Autodesk Inventor part; units mm, degrees
ref_plane "YZ Plane" through (0, 0, 0) normal (1, 0, 0) x (0, 1, 0)
ref_plane "XZ Plane" through (0, 0, 0) normal (0, 1, 0) x (-1, 0, 0)
ref_plane "XY Plane" through (0, 0, 0) normal (0, 0, 1) x (1, 0, 0)
sketch "Sketch1" plane through (0, 0, 0) normal (0, 0, 1) x (1, 0, 0)
  line L0 (0, 0) -> (139.7, 0)
  line L1 (139.7, 0) -> (139.7, 76.2)
  line L2 (139.7, 76.2) -> (0, 76.2)
  line L3 (0, 76.2) -> (0, 0)
  dimension "d0" = 139.7
  dimension "d1" = 76.2
extrude "Extrusion1" add sketch "Sketch1" along normal blind 3.175
sketch "Sketch2" plane through (0, 0, 3.175) normal (0, 0, 1) x (1, 0, 0)
  line L0 (0, 0) -> (139.7, 0)
  line L1 (139.7, 0) -> (139.7, 76.2)
  line L2 (139.7, 76.2) -> (0, 76.2)
  line L3 (0, 76.2) -> (0, 0)
  circle A0 centre (6.35, 69.85) radius 2.54
  circle A1 centre (6.35, 6.35) radius 2.54
  circle A2 centre (133.35, 6.35) radius 2.54
  circle A3 centre (133.35, 69.85) radius 2.54
  circle A4 centre (63.5, 38.1) radius 11.1125
  circle A5 centre (104.14, 38.1) radius 14.2875
  dimension "d4" = 6.35
  dimension "d5" = 6.35
  dimension "d6" = 69.85
  dimension "d7" = 6.35
  dimension "d8" = 133.35
  dimension "d9" = 6.35
  dimension "d10" = 133.35
  dimension "d11" = 69.85
  dimension "d12" = 63.5
  dimension "d13" = 38.1
  dimension "d14" = 38.1
  dimension "d15" = 104.14
  dimension "d16" = 5.08
  dimension "d17" = 5.08
  dimension "d18" = 5.08
  dimension "d19" = 5.08
  dimension "d20" = 22.225
  dimension "d21" = 28.575
extrude "Extrusion2" cut sketch "Sketch2" against normal blind 3.175 contours A0 | A1 | A2 | A3 | A4 | A5
sketch "Sketch3" plane through (0, 0, 3.175) normal (0, 0, 1) x (1, 0, 0)
  circle A0 centre (63.5, 38.1) radius 11.1125
  circle A1 centre (133.35, 6.35) radius 2.54
  circle A2 centre (6.35, 69.85) radius 2.54
  circle A3 centre (6.35, 6.35) radius 2.54
  circle A4 centre (133.35, 69.85) radius 2.54
  circle A5 centre (104.14, 38.1) radius 14.2875
  line L0 (0, 0) -> (139.7, 0)
  line L1 (139.7, 0) -> (139.7, 76.2)
  line L2 (139.7, 76.2) -> (0, 76.2)
  line L3 (0, 76.2) -> (0, 0)
  line L4 (0, 76.2) -> (0, 0)
  line L5 (0, 25.4) -> (-25.4, 25.4)
  line L6 (-25.4, 25.4) -> (-25.4, 50.8)
  line L7 (-25.4, 50.8) -> (0, 50.8)
  line L8 (0, 50.8) -> (0, 25.4)
  line L9 (0, 76.2) -> (-25.4, 50.8)
  line L10 (-25.4, 25.4) -> (0, 0)
  line L11 (139.7, 0) -> (139.7, 76.2)
  line L12 (139.7, 50.8) -> (165.1, 50.8)
  line L13 (165.1, 50.8) -> (165.1, 25.4)
  line L14 (165.1, 25.4) -> (139.7, 25.4)
  line L15 (139.7, 25.4) -> (139.7, 50.8)
  line L16 (0, 76.2) -> (0, 50.8)
  line L17 (0, 0) -> (0, 25.4)
  line L18 (139.7, 76.2) -> (139.7, 50.8)
  line L19 (165.1, 50.8) -> (139.7, 76.2)
  line L20 (165.1, 25.4) -> (139.7, 0)
  line L21 (139.7, 0) -> (139.7, 25.4)
  dimension "d24" = 25.4
  dimension "d25" = 25.4
  dimension "d26" = 25.4
  dimension "d27" = 25.4
  dimension "d28" = 25.4
  dimension "d29" = 25.4
extrude "Extrusion3" add sketch "Sketch3" against normal blind 3.175 contours L10 L5 L3 | L1 L14 L20 | L5 L6 L7 L3 | L1 L12 L13 L14 | L7 L9 L3 | L1 L19 L12
sketch "Sketch4" plane through (0, 0, 3.175) normal (0, 0, 1) x (1, 0, 0)
  circle A0 centre (63.5, 38.1) radius 11.1125
  circle A1 centre (133.35, 6.35) radius 2.54
  circle A2 centre (6.35, 69.85) radius 2.54
  circle A3 centre (6.35, 6.35) radius 2.54
  circle A4 centre (133.35, 69.85) radius 2.54
  circle A5 centre (104.14, 38.1) radius 14.2875
  line L0 (0, 0) -> (139.7, 0)
  line L1 (139.7, 0) -> (165.1, 25.4)
  line L2 (165.1, 25.4) -> (165.1, 50.8)
  line L3 (165.1, 50.8) -> (139.7, 76.2)
  line L4 (139.7, 76.2) -> (0, 76.2)
  line L5 (0, 76.2) -> (-25.4, 50.8)
  line L6 (-25.4, 50.8) -> (-25.4, 25.4)
  line L7 (-25.4, 25.4) -> (0, 0)
  circle A6 centre (-12.7, 38.1) radius 3.175
  circle A7 centre (152.4, 38.1) radius 3.175
  dimension "d32" = 6.35
  dimension "d33" = 12.7
  dimension "d34" = 38.1
  dimension "d35" = 6.35
  dimension "d36" = 152.4
  dimension "d37" = 38.1
extrude "Extrusion4" cut sketch "Sketch4" against normal blind 3.175 contours A6 | A7
properties part number "ToughBox Nano AM14U2 Mount" material "Aluminum 6061"
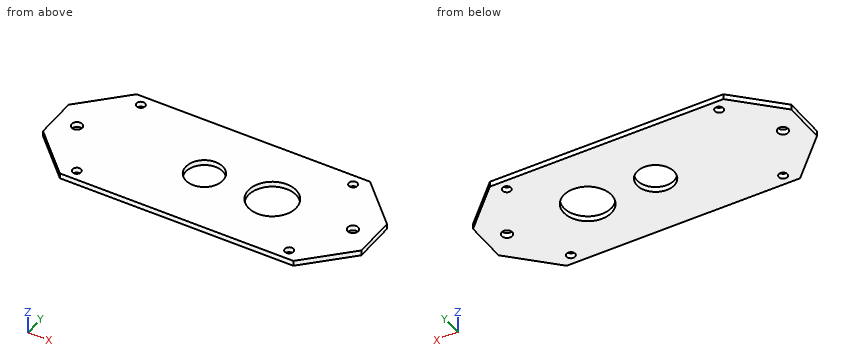
Part model, mm, in its own coordinate system. Round coordinates to 2 decimals unless told otherwise and drop trailing zeros. Write each loop counter-clockwise with the first axis right and the second up, starting at its lowest first coordinate (ties: lowest second). Pieces come first, ordered by that corner, then holes.
Item 1: Cut at D-D, the plane x = 63.5. Give the cut face in (y, z) (1 decimal), plus the area to 3 significant figures.
Results:
outline: (0, 0) - (27, 0) - (27, 3.2) - (0, 3.2) - close; (49.2, 0) - (76.2, 0) - (76.2, 3.2) - (49.2, 3.2) - close
area: 171 mm2
Item 2: Cut at A-A, the plane x = -12.7. Give the cut face in (y, z) (3 decimals), plus the area to 3 significant figures.
Results:
outline: (12.7, 0) - (34.925, 0) - (34.925, 3.175) - (12.7, 3.175) - close; (41.275, 0) - (63.5, 0) - (63.5, 3.175) - (41.275, 3.175) - close
area: 141 mm2
Item 3: Cut at C-C, the plane y = 69.85. Give the cut face in (x, z) (3 decimals), plus the area to 3 significant figures.
Results:
outline: (-6.35, 0) - (3.81, 0) - (3.81, 3.175) - (-6.35, 3.175) - close; (8.89, 0) - (130.81, 0) - (130.81, 3.175) - (8.89, 3.175) - close; (135.89, 0) - (146.05, 0) - (146.05, 3.175) - (135.89, 3.175) - close
area: 452 mm2
Item 4: Probe L1, parallel to Y at x = 6.35, z = 0.9; L2, parallel to Y at x = 64.5, z = 2.25; L3, parallel to X at y = 26.5, z = 2. List the from-to ranges inside material, lowest first.
Results:
L1: y = 0 to 3.81, 8.89 to 67.31, 72.39 to 76.2
L2: y = 0 to 27.03, 49.17 to 76.2
L3: x = -25.4 to 95.8, 112.48 to 165.1
Item 5: Cut at B-B, the plane z = 1.5. Count the separate pieces of the cut face and the enclosed holes in it, plus the area to 3 significant figures.
Results:
separate pieces: 1
enclosed holes: 8
area: 12,100 mm2
